from build123d import *

# Parameters (mm, degrees)
F0_W            = 127
F0_H            = 69.596
F1_DEPTH        = 19.05
F2_W            = 19.05
F2_H            = 69.596
F3_DEPTH        = 60.452
F4_R            = 19.05
F5_DEPTH        = 25.4
F7_DEPTH        = 25.4
F9_D            = 6.858
F9_DEPTH        = 25.4
F9_CSINK_D      = 10.16
F9_CSINK_ANGLE  = 82
F9_TIP          = 2.0603510626
F11_D           = 7.112
F11_DEPTH       = 25.4
F11_CBORE_D     = 12.7
F11_CBORE_DEPTH = 6.604
F11_TIP         = 2.1366603613


with BuildPart() as f1:
    # F0 (on Top) → F1 (new body)
    with BuildSketch(Plane.XY):
        Rectangle(F0_W, F0_H)
    extrude(amount=-F1_DEPTH)

    # F2 (on face) → F3 (join)
    with BuildSketch(Plane(origin=(0, 0, -19.05), x_dir=(1, 0, 0), z_dir=(0, 0, -1))):
        with Locations((-53.975, 0)):
            Rectangle(F2_W, F2_H)
    extrude(amount=F3_DEPTH)

    # F4 (on face) → F5 (cut)
    with BuildSketch(Plane.XY):
        Circle(F4_R)
    extrude(amount=-F5_DEPTH, mode=Mode.SUBTRACT)

    # F6 (on face) → F7 (cut)
    with BuildSketch(Plane.XY):
        with BuildLine():
            ThreePointArc((-3.1696624056, 27.2052425135), (0, 24.2142676058), (3.1696624056, 27.2052425135))
            ThreePointArc((3.1696624056, 27.2052425135), (0, 27.3892676058), (-3.1696624056, 27.2052425135))
        make_face()
        with BuildLine():
            ThreePointArc((-3.1696624056, 27.2052425135), (0, 27.3892676058), (3.1696624056, 27.2052425135))
            ThreePointArc((3.1696624056, 27.2052425135), (3.1736653209, 27.2972163639), (3.175, 27.3892676058))
            ThreePointArc((3.175, 27.3892676058), (-0.0920512419, 30.5629329266), (-3.1696624056, 27.2052425135))
        make_face()
        with BuildLine():
            ThreePointArc((27.2052425135, 3.1696624056), (27.3432226289, 1.5875), (27.3892676058, 0))
            ThreePointArc((27.3892676058, 0), (27.3432226289, -1.5875), (27.2052425135, -3.1696624056))
            ThreePointArc((27.2052425135, -3.1696624056), (29.568297818, -2.3092103269), (30.5642676058, 0))
            ThreePointArc((30.5642676058, 0), (29.568297818, 2.3092103269), (27.2052425135, 3.1696624056))
        make_face()
        with BuildLine():
            ThreePointArc((27.2052425135, -3.1696624056), (27.3432226289, -1.5875), (27.3892676058, 0))
            ThreePointArc((27.3892676058, 0), (27.3432226289, 1.5875), (27.2052425135, 3.1696624056))
            ThreePointArc((27.2052425135, 3.1696624056), (24.2142676058, 0), (27.2052425135, -3.1696624056))
        make_face()
        with BuildLine():
            ThreePointArc((3.175, -27.3892676058), (3.1736653209, -27.2972163639), (3.1696624056, -27.2052425135))
            ThreePointArc((3.1696624056, -27.2052425135), (0, -27.3892676058), (-3.1696624056, -27.2052425135))
            ThreePointArc((-3.1696624056, -27.2052425135), (-0.0920512419, -30.5629329266), (3.175, -27.3892676058))
        make_face()
        with BuildLine():
            ThreePointArc((-3.1696624056, -27.2052425135), (0, -27.3892676058), (3.1696624056, -27.2052425135))
            ThreePointArc((3.1696624056, -27.2052425135), (0, -24.2142676058), (-3.1696624056, -27.2052425135))
        make_face()
        with BuildLine():
            ThreePointArc((-24.2142676058, 0), (-25.0800572788, 2.1790302123), (-27.2052425135, 3.1696624056))
            ThreePointArc((-27.2052425135, 3.1696624056), (-27.3892676058, 0), (-27.2052425135, -3.1696624056))
            ThreePointArc((-27.2052425135, -3.1696624056), (-25.0800572788, -2.1790302123), (-24.2142676058, 0))
        make_face()
        with BuildLine():
            ThreePointArc((-27.2052425135, -3.1696624056), (-27.3892676058, 0), (-27.2052425135, 3.1696624056))
            ThreePointArc((-27.2052425135, 3.1696624056), (-30.5642676058, 0), (-27.2052425135, -3.1696624056))
        make_face()
    extrude(amount=-F7_DEPTH, mode=Mode.SUBTRACT)

    # F9
    with Locations(Plane.XY):
        with Locations((47.752, 19.05), (47.752, -19.05)):
            CounterSinkHole(F9_D / 2, F9_CSINK_D / 2, depth=F9_DEPTH, counter_sink_angle=F9_CSINK_ANGLE)
            with Locations((0, 0, -(F9_DEPTH + F9_TIP / 2))):  # 118° drill point
                Cone(0, F9_D / 2, F9_TIP, mode=Mode.SUBTRACT)

    # F11
    with Locations(Plane(origin=(-63.5, 0, 0), x_dir=(0, -1, 0), z_dir=(-1, 0, 0))):
        with Locations((-19.05, -63.754), (19.05, -63.754)):
            CounterBoreHole(F11_D / 2, F11_CBORE_D / 2, F11_CBORE_DEPTH, depth=F11_DEPTH)
            with Locations((0, 0, -(F11_DEPTH + F11_TIP / 2))):  # 118° drill point
                Cone(0, F11_D / 2, F11_TIP, mode=Mode.SUBTRACT)


solid = f1.part
For this review, take the finished solid that the model builds, in its own axes (mm). A direction names the side the tool comes from. Give positions to 0.01 mm unless a question says otherwise; leave off trailing zeros. Order: outer loops, then holes, each group sorted by start corner. A loop starts at its lowest first (then second) coordinate and runs counter-clockwise, first axis right, second up. Notation, with made-up numbers: M -12.5,4.25 L -2.5,4.25 A18 ccw -2.5,10.25 Z; hole C 51.25,-25.5 d1. An arc over 180 degrees is marked long. Answer in a Markdown table with one row per item. Add a question column.
(1) Consider section D-D on x = 15. State the section outline as (y, z) points.
(2) Wall thickness on probe 1 along Y at (x, z) = (0, -11); probe 2 along X at (y, z) = (-27.5, -5); probe 3 along X at (y, z) = (-17, -7): over which ranges is each line inside the solid? List them lowest first. Write a range as [from, to].
(3) For pin 1 (11.5 mm diameter, centred on y = -19.05, z = -63.754, fed in from -X); pin 2 (7.5 mm diameter, centred on y = 19.05, z = -63.754, fed in from +X); pin 3 (11 mm diameter, centred on x = 47.752, y = -19.05, fed in from -Z), all flat-tipped, find the tip position at first contact; note any pin that passes through.
(4) Mouldability with a two-part tool opening along X and no side actions: class faces 4 (the face through (44.6, 17.7, -10.6)), 5 (the face through (-54, 0, -79.502)), 6 (the face through (-56.896, -22, -66)) as +X half, -X half, draft (parallel to the pull), parting line (faces both ways), or undercut.
(5) Consider section A-A on x = 0. State the section outline as (y, z) points.
(6) Consider section C-C on z = -15.5. State the section outline as (x, y) points (3 decimals).
(7) For faces 1 (the face through (-60.244, -25.107, -61.847)), 2 (the face through (-44.45, 0, -49)), 3 (the face through (-63.5, 0, -39)), list the 3-axis set-ups (+Z, -Z, +X, -X, +Y, -Y) from which the entire face can be reached by the end or side of a thin tool; tool diameter is ignored.
(8) Consider section B-B on y = -8.5. State the section outline as (x, z) points.
Evaluation:
| question | item | result |
|---|---|---|
| 1 | outline | M -34.8,-19.05 L -11.74,-19.05 L -11.74,0 L -34.8,0 Z; M 11.74,-19.05 L 34.8,-19.05 L 34.8,0 L 11.74,0 Z |
| 2 | probe 1 | y = [-34.8, -30.56], [-24.21, -19.05], [19.05, 24.21], [30.56, 34.8] |
| 2 | probe 2 | x = [-63.5, -3.17], [3.17, 63.5] |
| 2 | probe 3 | x = [-63.5, -8.6], [8.6, 45], [50.5, 63.5] |
| 3 | pin 1 | stops at x = -56.9 |
| 3 | pin 2 | stops at x = -44.45 |
| 3 | pin 3 | stops at z = -19.05 |
| 4 | face 4 | undercut |
| 4 | face 5 | draft |
| 4 | face 6 | -X half |
| 5 | outline | M -34.8,-19.05 L -30.56,-19.05 L -30.56,0 L -34.8,0 Z; M -24.21,-19.05 L -19.05,-19.05 L -19.05,0 L -24.21,0 Z; M 19.05,-19.05 L 24.21,-19.05 L 24.21,0 L 19.05,0 Z; M 30.56,-19.05 L 34.8,-19.05 L 34.8,0 L 30.56,0 Z |
| 6 | outline | M -63.5,-34.798 L 63.5,-34.798 L 63.5,34.798 L -63.5,34.798 Z; hole C -27.389,0 d6.35; hole C 0,0 d38.1; hole C 0,-27.389 d6.35; hole C 0,27.389 d6.35; hole C 27.389,0 d6.35; hole C 47.752,-19.05 d6.858; hole C 47.752,19.05 d6.858 |
| 7 | face 1 | -X |
| 7 | face 2 | -Z, +X, +Y, -Y |
| 7 | face 3 | +Z, -Z, -X, +Y, -Y |
| 8 | outline | M -63.5,-79.5 L -44.45,-79.5 L -44.45,-19.05 L -17.05,-19.05 L -17.05,0 L -63.5,0 Z; M 17.05,-19.05 L 63.5,-19.05 L 63.5,0 L 17.05,0 Z |
